Source: CAD feature listing. Evaluate the final solid. Frame: model axes, mm. Round coordinates to 2 decimals unless told otherwise and drop trailing zeros. Loops run counter-clockwise (first coordinate to the right, second up) from the corner with the lowest first, then second, coordinate; pieces in that order, holes last. Notation, with made-up numbers: (64, 6.5) - (81, 6.5) arc R22 ccw to (81, 15.5) - close; hole circle Ø6 at (-40, 18.5). An arc over 180 degrees is marked (long way). One line per question, with ' | ' between items.
Autodesk Inventor part; units mm, degrees
ref_plane "YZ Plane" through (0, 0, 0) normal (1, 0, 0) x (0, 1, 0)
ref_plane "XZ Plane" through (0, 0, 0) normal (0, 1, 0) x (-1, 0, 0)
ref_plane "XY Plane" through (0, 0, 0) normal (0, 0, 1) x (1, 0, 0)
sketch "Sketch1" plane through (0, 0, 0) normal (0, 0, 1) x (1, 0, 0)
  line L0 (0, 0) -> (400, 0)
  line L1 (400, 0) -> (400, 100)
  line L2 (400, 100) -> (0, 100)
  line L3 (0, 100) -> (0, 0)
  circle A0 centre (0, 50) radius 50
  circle A1 centre (400, 50) radius 50
  dimension "d0" = 400
  dimension "d1" = 100
extrude "Extrusion1" add sketch "Sketch1" along normal blind 10
sketch "Sketch2" plane through (0, 0, 10) normal (0, 0, 1) x (1, 0, 0)
  arc A0 (0, 100) -> (0, 0) centre (0, 50) ccw
  arc A1 (400, 0) -> (400, 100) centre (400, 50) ccw
hole "Hole1" at (0, 50, 10) at (400, 50, 10) direction (0, 0, -1) diameter 8 end through all
sketch "Sketch3" plane through (0, 0, 10) normal (0, 0, 1) x (1, 0, 0)
  circle A0 centre (0, 50) radius 4
  circle A1 centre (400, 50) radius 4
  point P0 (125, 50)
  point P1 (275, 51.5)
  dimension "d11" = 125
  dimension "d55" = 125
hole "Hole2" at (125, 50, 10) at (275, 51.5, 10) direction (0, 0, -1) diameter 16 end through all
sketch "Sketch4" plane through (0, 0, 10) normal (0, 0, 1) x (1, 0, 0)
  circle A0 centre (275, 51.5) radius 8
  circle A1 centre (125, 50) radius 8
  line L0 (110, 65) -> (140, 65)
  line L1 (140, 65) -> (140, 35)
  line L2 (140, 35) -> (110, 35)
  line L3 (110, 35) -> (110, 65)
  line L4 (260, 66.5) -> (290, 66.5)
  line L5 (290, 66.5) -> (290, 36.5)
  line L6 (290, 36.5) -> (260, 36.5)
  line L7 (260, 36.5) -> (260, 66.5)
  dimension "d22" = 30
  dimension "d23" = 30
  dimension "d26" = 30
  dimension "d27" = 30
  dimension "d30" = 15
  dimension "d32" = 15
  dimension "d34" = 15
  dimension "d36" = 15
hole "Hole3" at (110, 35, 10) at (110, 65, 10) at (140, 65, 10) at (140, 35, 10) at (260, 36.5, 10) at (260, 66.5, 10) at (290, 66.5, 10) at (290, 36.5, 10) direction (0, 0, -1) diameter 4 end through all
sketch "Sketch5" plane through (0, 0, 10) normal (0, 0, 1) x (1, 0, 0)
  circle A0 centre (140, 35) radius 2
  circle A1 centre (140, 65) radius 2
  circle A2 centre (110, 65) radius 2
  circle A3 centre (110, 35) radius 2
  circle A4 centre (125, 50) radius 8
  line L0 (105, 70) -> (145, 70)
  line L1 (145, 70) -> (145, 30)
  line L2 (145, 30) -> (105, 30)
  line L3 (105, 30) -> (105, 70)
  circle A5 centre (275, 51.5) radius 8
  line L4 (255, 71.5) -> (295, 71.5)
  line L5 (295, 71.5) -> (295, 31.5)
  line L6 (295, 31.5) -> (255, 31.5)
  line L7 (255, 31.5) -> (255, 71.5)
  dimension "d45" = 40
  dimension "d46" = 40
  dimension "d47" = 20
  dimension "d48" = 20
  dimension "d51" = 40
  dimension "d52" = 40
  dimension "d53" = 20
  dimension "d54" = 20
extrude "Extrusion2" cut sketch "Sketch5" against normal blind 5
equation "\"d32\" = d30"
equation "\"d36\" = d34"
properties part number "base side"
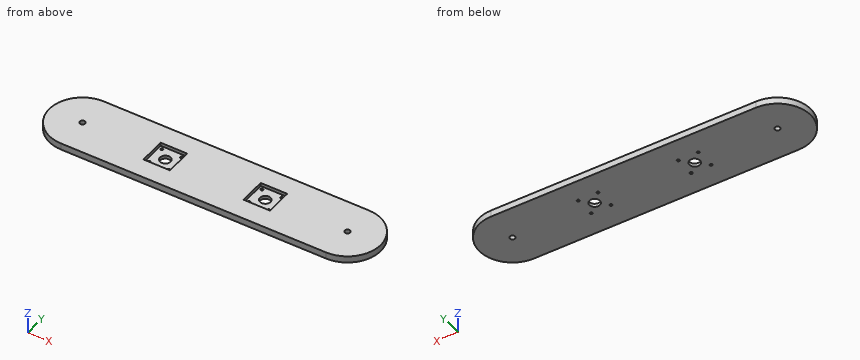
1. Section query B-B, the plane x = 125. Return loops of the section in (y, z).
Worked out:
outline: (0, 0) - (42, 0) - (42, 5) - (30, 5) - (30, 10) - (0, 10) - close; (58, 0) - (100, 0) - (100, 10) - (70, 10) - (70, 5) - (58, 5) - close
2. Contact query for flat-ended pins moving along their axis: P1, Ø5.5, axis at y = 44, z = 6.5, coming from the -X side; P2, Ø2, axis at y = 25, z = 3, coming from the +X side; P3, Ø2.5, axis at y = 49, z = 6.5, coming from the -X side; P4, Ø3.5, axis at x = 290, y = 36.5, coming from the +Z side. Output: stop coordinate, or through.
Worked out:
P1: stops at x = -49.89 | P2: stops at x = 443.86 | P3: stops at x = -50 | P4: passes through
3. Section query A-A, the plane z = 8.25. Return loops of the section in (x, y).
Worked out:
outline: (0, 0) - (400, 0) arc R50 ccw to (400, 100) - (0, 100) arc R50 ccw to start; hole circle Ø8 at (0, 50); hole (105, 30) - (145, 30) - (145, 70) - (105, 70) - close; hole (255, 31.5) - (295, 31.5) - (295, 71.5) - (255, 71.5) - close; hole circle Ø8 at (400, 50)
4. Material intervals for probe 1 along Y at (x, z) = (290, 1.15); probe 2 along Y at (x, z) = (110, 1.1); probe 3 along Y at (x, z) = (400, 6.25), sorted ascending.
Worked out:
probe 1: y = 0 to 34.5, 38.5 to 64.5, 68.5 to 100 | probe 2: y = 0 to 33, 37 to 63, 67 to 100 | probe 3: y = 0 to 46, 54 to 100
5. Section query C-C, the plane y = 91. Return loops of the section in (x, z).
Worked out:
outline: (-28.62, 0) - (428.62, 0) - (428.62, 10) - (-28.62, 10) - close
